from build123d import *

# Parameters (mm, degrees)
ESQUISSE1_W             = 50
ESQUISSE1_H             = 10
BOSS_EXTRU_1_DEPTH      = 10
ENL_V_MAT_EXTRU_1_DEPTH = 10
ESQUISSE3_R             = 2
BOSS_EXTRU_2_DEPTH      = 5
ENL_V_MAT_EXTRU_2_DEPTH = 52.961524227
ESQUISSE6_R             = 2
BOSS_EXTRU_3_DEPTH      = 5


with BuildPart() as part:
    # Esquisse1 → Boss.-Extru.1 (new body)
    with BuildSketch(Plane(origin=(0, 0, 0), x_dir=(1, 0, 0), z_dir=(0, 1, 0))):
        with Locations((25, 5)):
            Rectangle(ESQUISSE1_W, ESQUISSE1_H)
    extrude(amount=BOSS_EXTRU_1_DEPTH)

    # Esquisse2 → Enl_v. mat.-Extru.1 (cut)
    with BuildSketch(Plane.XY):
        Polygon((0, 3), (20, 3), (30, 3), (50, 3), (50, 7), (30, 7), (20, 7), (0, 7), align=None)
    extrude(amount=-ENL_V_MAT_EXTRU_1_DEPTH, mode=Mode.SUBTRACT)


with BuildPart() as enl_v_mat_extru_1_piece_1:
    # of the separate pieces the step leaves, piece 1, a body of its own (enl_v_mat_extru_1_pieces)
    add(part.part.solids().sort_by_distance((0, 7, 0))[0])

    # Esquisse3 → Boss.-Extru.2 (add)
    with BuildSketch(Plane(origin=(0, 3, 0), x_dir=(1, 0, 0), z_dir=(0, 1, 0))):
        with Locations(Location((5, 5, 0), (0, 0, 270))):
            Circle(ESQUISSE3_R)
        with Locations(Location((45, 5, 0), (0, 0, 270))):
            Circle(ESQUISSE3_R)
    extrude(amount=BOSS_EXTRU_2_DEPTH)


with BuildPart() as enl_v_mat_extru_1_piece_2:
    # of the separate pieces the step leaves, piece 2, a body of its own (enl_v_mat_extru_1_pieces)
    add(part.part.solids().sort_by_distance((0, 0, 0))[0])


with BuildPart() as enl_v_mat_extru_2_tool:
    # Esquisse4 → Enl_v. mat.-Extru.2 (new, through all)
    with BuildSketch(Plane(origin=(0, 10, 0), x_dir=(1, 0, 0), z_dir=(0, 1, 0))):
        with BuildLine():
            Line((5, 0), (-6.304307012, 0))
            Line((-6.304307012, 0), (-6.304307012, 10))
            Line((-6.304307012, 10), (5, 10))
            ThreePointArc((5, 10), (0, 5), (5, 0))
        make_face()
        with BuildLine():
            Line((45, 0), (61.280681511, 0))
            Line((61.280681511, 0), (61.280681511, 10))
            Line((61.280681511, 10), (45, 10))
            ThreePointArc((45, 10), (50, 5), (45, 0))
        make_face()
    extrude(amount=-ENL_V_MAT_EXTRU_2_DEPTH)


with BuildPart() as enl_v_mat_extru_1_piece_1_1:
    add(enl_v_mat_extru_1_piece_1.part)

    # Enl_v. mat.-Extru.2: cut by enl_v_mat_extru_2_tool
    add(enl_v_mat_extru_2_tool.part, mode=Mode.SUBTRACT)



with BuildPart() as enl_v_mat_extru_1_piece_2_1:
    add(enl_v_mat_extru_1_piece_2.part)

    # Enl_v. mat.-Extru.2: cut by enl_v_mat_extru_2_tool
    add(enl_v_mat_extru_2_tool.part, mode=Mode.SUBTRACT)


with BuildPart() as enl_v_mat_extru_1_piece_1_2:
    add(enl_v_mat_extru_1_piece_1_1.part)

    add(enl_v_mat_extru_1_piece_2_1.part)  # Boss.-Extru.3 merges Enl_v. mat.-Extru.1 piece 2
    # Esquisse6 → Boss.-Extru.3 (add)
    with BuildSketch(Plane.XZ.offset(-7)):
        with Locations(Location((21, -5, 0), (0, 0, 90))):
            Circle(ESQUISSE6_R)
    extrude(amount=BOSS_EXTRU_3_DEPTH)


solid = enl_v_mat_extru_1_piece_1_2.part
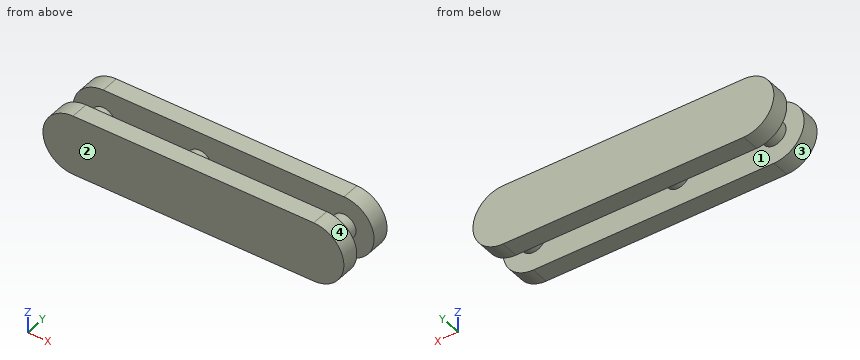
Geometry check sheet. Reference: the model listing, model coordinates, mm. Face numbers are marked on the shaded views. Coordinates: 2 decimals unless noted, no trailing zeros. Write each loop counter-clockwise with the first axis right and the second up, starting at its lowest first coordinate (ties: lowest second). Pieces come first, ordered by that corner, then holes. Notation, with made-up numbers: (84, 12.5) -> (116, 12.5) arc R26 ccw to (116, 48.5) -> close; hole circle Ø3 at (-35, 61). An arc over 180 degrees is marked (long way). One line per question, with ' | ' between items.
1. Cross-section at C-C on y = 6. Record the cut outline in (x, z).
Answers:
outline: circle Ø4 at (5, -5); circle Ø4 at (21, -5); circle Ø4 at (45, -5)
2. Draft check along X on the marked faces 1, 2, 3 and 4. Enter one of: +X half, -X half, draft (parallel to the pull), parting line (faces both ways), or undercut.
Answers:
face 1: undercut | face 2: draft | face 3: -X half | face 4: +X half
3. Cross-section at B-B on z = -5. Record the cut outline in (x, y), and give its area (3 significant figures).
Answers:
outline: (0, 0) -> (50, 0) -> (50, 3) -> (47, 3) -> (47, 7) -> (50, 7) -> (50, 10) -> (0, 10) -> (0, 7) -> (3, 7) -> (3, 3) -> (0, 3) -> close; hole (7, 3) -> (19, 3) -> (19, 7) -> (7, 7) -> close; hole (23, 3) -> (43, 3) -> (43, 7) -> (23, 7) -> close | area: 348 mm²
4. Thickness scan on probe 1 along Y at (x, z) = (35.5, -4.5); probe 2 along Z at (x, y) = (45, 5.25); probe 3 along X at (y, z) = (7.25, -3.75). Record the ranges inside material, lowest first. Write a range as from..to.
Answers:
probe 1: y = 0..3, 7..10 | probe 2: z = -7..-3 | probe 3: x = 0.16..49.84
5. Depth check by flat-ended pin: pin 1 Ø6 at (y, z) = (4, -8.5) entering from -X. Enter the tip coordinate at first touch or a pass-through.
Answers:
pin 1: stops at x = 0.05
6. Cross-section at A-A on x = 12. Record the cut outline in (y, z), and give its area (3 significant figures).
Answers:
outline: (0, -10) -> (3, -10) -> (3, 0) -> (0, 0) -> close; (7, -10) -> (10, -10) -> (10, 0) -> (7, 0) -> close | area: 60.0 mm²
7. Cross-section at D-D on x = 21. Record the cut outline in (y, z).
Answers:
outline: (0, -10) -> (3, -10) -> (3, -7) -> (7, -7) -> (7, -10) -> (10, -10) -> (10, 0) -> (7, 0) -> (7, -3) -> (3, -3) -> (3, 0) -> (0, 0) -> close
